```python
from build123d import *

# Parameters (mm, degrees)
SKETCH1_W           = 40
SKETCH1_H           = 3
BOSS_EXTRUDE1_DEPTH = 3
SKETCH2_R           = 1.25
CUT_EXTRUDE1_DEPTH  = 10
SKETCH3_W           = 16
SKETCH3_H           = 3
SKETCH3_W_2         = 11
SKETCH3_H_2         = 2.000440009
CUT_EXTRUDE2_DEPTH  = 10


with BuildPart() as part:
    # Sketch1 → Boss-Extrude1 (new body)
    with BuildSketch(Plane(origin=(0, 0, 0), x_dir=(1, 0, 0), z_dir=(0, 1, 0))):
        Polygon((20, 37.5), (20, 12.5), (0, 12.5), (0, 0), (10, 0), (10, -16), (70, -16), (70, 0), (80, 0), (80, 12.5), (60, 12.5), (60, 37.5), (80, 37.5), (80, 50), (70, 50), (70, 66), (10, 66), (10, 50), (0, 50), (0, 37.5), align=None)
        with Locations((40, -4.5)):
            Rectangle(SKETCH1_W, SKETCH1_H, mode=Mode.SUBTRACT)
        with Locations((40, 54.5)):
            Rectangle(SKETCH1_W, SKETCH1_H, mode=Mode.SUBTRACT)
    extrude(amount=BOSS_EXTRUDE1_DEPTH)

    # Sketch2 → Cut-Extrude1 (cut)
    with BuildSketch(Plane(origin=(0, 0, 0), x_dir=(1, 0, 0), z_dir=(0, 1, 0))):
        with Locations(Location((31.25, -11, 0), (0, 0, 270))):
            Circle(SKETCH2_R)
        with Locations(Location((48.75, -11, 0), (0, 0, 270))):
            Circle(SKETCH2_R)
    extrude(amount=CUT_EXTRUDE1_DEPTH, mode=Mode.SUBTRACT)

    # Sketch3 → Cut-Extrude2 (cut)
    with BuildSketch(Plane(origin=(0, 0, 0), x_dir=(1, 0, 0), z_dir=(0, 1, 0))):
        with Locations((18, -14.5)):
            Rectangle(SKETCH3_W, SKETCH3_H)
        Polygon((37, -16), (40, -16), (40, -11), (37, -11), (37, -13.999559991), align=None)
        Polygon((40, -11), (40, -16), (43, -16), (43, -13.999559991), (43, -11), align=None)
        with Locations((62, -14.5)):
            Rectangle(SKETCH3_W, SKETCH3_H)
        with Locations((31.5, -14.999779996)):
            Rectangle(SKETCH3_W_2, SKETCH3_H_2)
        with Locations((48.5, -14.999779996)):
            Rectangle(SKETCH3_W_2, SKETCH3_H_2)
    extrude(amount=CUT_EXTRUDE2_DEPTH, mode=Mode.SUBTRACT)


solid = part.part
```
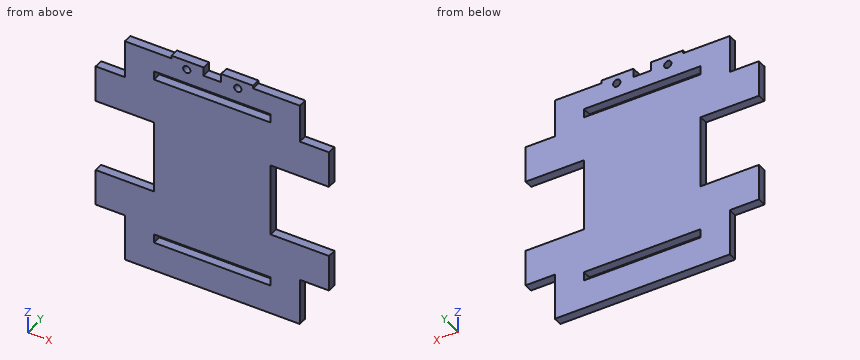
Input: part model. Units: mm. Frame: model coordinates. Coordinates: 2 decimals unless noted, no trailing zeros. Loops run counter-clockwise (first coordinate to the right, second up) from the corner with the lowest first, then second, coordinate; pieces in that order, holes last. Notation, with made-up numbers: (70.5, -40) - (105.5, -40) arc R18 cw to (105.5, -30) - close; hole circle Ø7 at (62.25, 76.25). An arc over 180 degrees is marked (long way). Answer in a Markdown table with one row per item.
(1) Cut plane B-B on x = 48.75. Output: boundary loops of the cut face in (y, z).
Model answer:
| item | result |
|---|---|
| outline | (0, -66) - (3, -66) - (3, -56) - (0, -56) - close; (0, -53) - (3, -53) - (3, 3) - (0, 3) - close; (0, 6) - (3, 6) - (3, 9.75) - (0, 9.75) - close; (0, 12.25) - (3, 12.25) - (3, 14) - (0, 14) - close |
(2) Pin query (flat end, axial travel): P1, Ø0.9, axis at y = 1, z = -61.5, coming from the -X side; P2, Ø1.5, axis at y = 2, z = -23, coming from the +X side; P3, Ø4, axis at x = 30.5, z = -38, coming from the -Y side; P4, Ø0.8, axis at y = 1, z = 13.5, coming from the +X side. Return the tip coordinate at first contact, or that it passes through.
Model answer:
| item | result |
|---|---|
| P1 | stops at x = 10 |
| P2 | stops at x = 60 |
| P3 | stops at y = 0 |
| P4 | stops at x = 54 |
(3) Cut plane C-C on x = 38. Output: boundary loops of the cut face in (y, z), plus the area to 3 significant figures.
Model answer:
| item | result |
|---|---|
| outline | (0, -66) - (3, -66) - (3, -56) - (0, -56) - close; (0, -53) - (3, -53) - (3, 3) - (0, 3) - close; (0, 6) - (3, 6) - (3, 11) - (0, 11) - close |
| area | 213 mm² |
(4) Material intervals for L1, parallel to Z at x = 31.25, y = 2.35; L2, parallel to Z at x = 50.5, y = 2.5; L3, parallel to Z at x = 42.5, y = 2.3, sorted ascending. Write a range as from..to.
Model answer:
| item | result |
|---|---|
| L1 | z = -66..-56, -53..3, 6..9.75, 12.25..14 |
| L2 | z = -66..-56, -53..3, 6..14 |
| L3 | z = -66..-56, -53..3, 6..11 |
(5) Cut plane D-D on x = 18. Output: boundary loops of the cut face in (y, z).
Model answer:
| item | result |
|---|---|
| outline | (0, -66) - (3, -66) - (3, -37.5) - (0, -37.5) - close; (0, -12.5) - (3, -12.5) - (3, 13) - (0, 13) - close |
(6) Cut plane A-A on x = 73.5. Output: boundary loops of the cut face in (y, z), plus the area to 3 significant figures.
Model answer:
| item | result |
|---|---|
| outline | (0, -50) - (3, -50) - (3, -37.5) - (0, -37.5) - close; (0, -12.5) - (3, -12.5) - (3, 0) - (0, 0) - close |
| area | 75.0 mm² |
